For this review, take the finished solid that the model builds, in its own axes (mm). Give positions to 0.01 mm unless a question says otherwise; leave off trailing zeros. Loops run counter-clockwise (first coordinate to the right, second up) from the corner with the lowest first, then second, coordinate; pieces in that order, holes last. Notation, with made-up numbers: (28, 34) - (71, 34) arc R25 cw to (71, 68) - close; hole circle Ø3 at (81.25, 9). An arc over 180 degrees is marked (long way). Put each result on its own line as item: value. Start each with the question number.
from build123d import *

# Parameters (mm, degrees)
SKETCH_1_R          = 101.5
EXTRUDE_1_DEPTH     = 54
FILLET_1_R          = 10
SKETCH_2_R          = 6
CUT_EXTRUDE_1_DEPTH = 54


with BuildPart() as part:
    # 草圖1 → 填料-伸長1 (new body)
    with BuildSketch(Plane.XY):
        Circle(SKETCH_1_R)
    extrude(amount=EXTRUDE_1_DEPTH)

    # 圓角1
    fillet_1_edges = [part.edges().sort_by_distance(p)[0] for p in [
        (-101.5, 0, 0),
        (-101.5, 0, 54),
    ]]
    fillet(fillet_1_edges, radius=FILLET_1_R)

    # 草圖2 → 除料-伸長1 (cut)
    with BuildSketch(Plane(origin=(0, 0, 0), x_dir=(-1, 0, 0), z_dir=(0, 0, -1))):
        Circle(SKETCH_2_R)
    extrude(amount=-CUT_EXTRUDE_1_DEPTH, mode=Mode.SUBTRACT)


solid = part.part
1) Take a section at C-C on z = 29.5. State the section outline as (x, y) points.
2) Take a section at A-A on x = 0. State the section outline as (y, z) points.
3) Wall thickness on probe 1 along Y at (x, z) = (0, 21); probe 2 along Y at (x, z) = (-46, 25); probe 3 along X at (y, z) = (44.5, 34.5) (3 decimals): over which ranges is each line inside the solid? List them lowest first.
4) Take a section at D-D on z = 46.5. State the section outline as (x, y) points.
5) Mouldability with a two-part tool opening along X and no side actions: class faces 1 (the cylindrical face through (6, 0, 27)), 2 (the flat face through (-1, -19, 54)), 3 (the cylindrical face through (96.813, 30.488, 26.762)) as released by +X, released by -X, zero draft, split by the parting line, or undercut.
6) Insertion check: P1, Ø1.5, axis at x = 25, z = 40, coming from the -Y side; P2, Ø4, axis at y = 55.5, z = 18.5, coming from the +X side; P3, Ø8, axis at y = 24.5, z = 12.5, coming from the +X side; P4, Ø19, axis at x = 0, y = 0, coming from the +Z side. Each pin has a flat end and moves straight along its axis. Give the tip position at first contact, or say it passes through.
Answers follow:
1. outline: circle Ø203 at (0, 0); hole circle Ø12 at (0, 0)
2. outline: (-101.5, 10) arc R10 ccw to (-91.5, 0) - (-6, 0) - (-6, 54) - (-91.5, 54) arc R10 ccw to (-101.5, 44) - close; (6, 0) - (91.5, 0) arc R10 ccw to (101.5, 10) - (101.5, 44) arc R10 ccw to (91.5, 54) - (6, 54) - close
3. probe 1: -101.5 to -6, 6 to 101.5
3. probe 2: -90.48 to 90.48
3. probe 3: -91.225 to 91.225
4. outline: circle Ø202.36 at (0, 0); hole circle Ø12 at (0, 0)
5. face 1: undercut
5. face 2: zero draft
5. face 3: split by the parting line
6. P1: y = -98.56
6. P2: x = 86.26
6. P3: x = 99.41
6. P4: z = 54
